```python
from build123d import *

# Parameters (mm, degrees)
SKETCH_W  = 80
SKETCH_H  = 10
SKETCH_R  = 1.5
PAD_DEPTH = 3
FILLET_R  = 0.5


with BuildPart() as part:
    # Sketch → Pad (new body)
    with BuildSketch(Plane.XY):
        Rectangle(SKETCH_W, SKETCH_H)
        with Locations((-32, 0)):
            Circle(SKETCH_R, mode=Mode.SUBTRACT)
        with Locations((-24, 0)):
            Circle(SKETCH_R, mode=Mode.SUBTRACT)
        with Locations((-8, 0)):
            Circle(SKETCH_R, mode=Mode.SUBTRACT)
        Circle(SKETCH_R, mode=Mode.SUBTRACT)
        with Locations((8, 0)):
            Circle(SKETCH_R, mode=Mode.SUBTRACT)
        with Locations((16, 0)):
            Circle(SKETCH_R, mode=Mode.SUBTRACT)
        with Locations((24, 0)):
            Circle(SKETCH_R, mode=Mode.SUBTRACT)
        with Locations((32, 0)):
            Circle(SKETCH_R, mode=Mode.SUBTRACT)
        with Locations((-16, 0)):
            Circle(SKETCH_R, mode=Mode.SUBTRACT)
    extrude(amount=PAD_DEPTH)

    # Fillet
    fillet_edges = [part.edges().sort_by_distance(p)[0] for p in [
        (-40, 5, 1.5),
        (-40, -5, 1.5),
        (-40, 0, 3),
        (-40, 0, 0),
        (0, 5, 3),
        (0, 5, 0),
        (0, -5, 3),
        (40, 0, 3),
        (40, 5, 1.5),
        (40, 0, 0),
        (40, -5, 1.5),
        (0, -5, 0),
    ]]
    fillet(fillet_edges, radius=FILLET_R)


solid = part.part
```
Check sheet for the modelled part. Datum: model origin and axes. Units: mm. Give positions to 0.01 mm unless a question says otherwise; leave off trailing zeros. Write each loop counter-clockwise with the first axis right and the second up, starting at its lowest first coordinate (ties: lowest second). Pieces come first, ordered by that corner, then holes.
Item 1: Scan lines: L1, parallel to Y at x = 16, z = 1.5; L2, parallel to Y at x = -17, z = 1.25; L3, parallel to Y at x = 30, z = 0.2. Record each from-to range of solid material in increasing order.
Item 2: Cross-section at B-B (z = 1.1). Count the separate pieces of the cut face and the enclosed holes in it, and give its area (3 significant figures).
Item 3: Cross-section at A-A (x = -16). Enter the section's corners in (y, z).
Item 4: Draft check along X on faces 1 (the face through (-1, 5, 1)), 2 (the face through (-9.5, 0.07, 1.48)), 3 (the face through (-40, 0, 1)). Enter one of: released by +X, released by -X, zero draft, split by the parting line, or undercut.
Report:
1. L1: y = -5 to -1.5, 1.5 to 5
1. L2: y = -5 to -1.12, 1.12 to 5
1. L3: y = -4.9 to 4.9
2. separate pieces: 1
2. enclosed holes: 9
2. area: 736 mm2
3. outline: (-5, 0.5) arc R0.5 ccw to (-4.5, 0) - (-1.5, 0) - (-1.5, 3) - (-4.5, 3) arc R0.5 ccw to (-5, 2.5) - close; (1.5, 0) - (4.5, 0) arc R0.5 ccw to (5, 0.5) - (5, 2.5) arc R0.5 ccw to (4.5, 3) - (1.5, 3) - close
4. face 1: zero draft
4. face 2: undercut
4. face 3: released by -X
